The model under review builds one solid part; all positions refer to its coordinate system, in mm. A direction names the side the tool comes from. Round coordinates to 2 decimals unless told otherwise and drop trailing zeros. One line per item, written item: value. Start each with the question number.
1) Mouldability with a two-part tool opening along Y and no side actions: class faces 1 (the face through (-84.437, -39.217, 4.986)), 2 (the face through (-1, 1, 6)), 3 (the face through (-1, -75, 3)) as +Y half, -Y half, draft (parallel to the pull), parting line (faces both ways), or undercut.
2) Tool access review of faces 4 (the face through (84.73, -35.05, 1.97)), 5 (the face through (-84.437, 36.783, 4.986)): name each direction out of +Z, -Z, +X, -X, +Y, -Y from which nothing blocks a thin tool from reaching the whole face with its end or side.
3) Wall thickness on probe 1 along Y at (x, z) = (-82.85, 1.05); probe 2 along Y at (x, z) = (82.85, 4.5): over which ranges is each line inside the solid? List them lowest first.
4) For P1, Ø3.5, axis at x = -82, y = -37.5, coming from the -Z side, flat-tipped, find the tip position at first contact; note if it passes through.
from build123d import *

# Parameters (mm, degrees)
F0_W     = 200
F0_H     = 150
F0_R     = 3.5
F0_R_2   = 2
F1_DEPTH = 6
F2_DEPTH = 4


with BuildPart() as f1:
    # F0 (on Top) → F1 (new body)
    with BuildSketch(Plane.XY):
        Rectangle(F0_W, F0_H)
        with Locations((-82.85, -38)):
            Circle(F0_R, mode=Mode.SUBTRACT)
        with Locations((82.85, -38)):
            Circle(F0_R, mode=Mode.SUBTRACT)
        with Locations((-82.85, 38)):
            Circle(F0_R, mode=Mode.SUBTRACT)
        with Locations((82.85, 38)):
            Circle(F0_R, mode=Mode.SUBTRACT)
        with Locations((-82.85, 38)):
            Circle(F0_R)
        with Locations((-82.85, 38)):
            Circle(F0_R_2, mode=Mode.SUBTRACT)
        with Locations((82.85, -38)):
            Circle(F0_R)
        with Locations((82.85, -38)):
            Circle(F0_R_2, mode=Mode.SUBTRACT)
        with Locations((82.85, 38)):
            Circle(F0_R)
        with Locations((82.85, 38)):
            Circle(F0_R_2, mode=Mode.SUBTRACT)
        with Locations((-82.85, -38)):
            Circle(F0_R)
        with Locations((-82.85, -38)):
            Circle(F0_R_2, mode=Mode.SUBTRACT)
    extrude(amount=F1_DEPTH)

    # F0 (on Top) → F2 (cut)
    with BuildSketch(Plane.XY):
        with Locations((-82.85, 38)):
            Circle(F0_R)
        with Locations((-82.85, 38)):
            Circle(F0_R_2, mode=Mode.SUBTRACT)
        with Locations((82.85, 38)):
            Circle(F0_R)
        with Locations((82.85, 38)):
            Circle(F0_R_2, mode=Mode.SUBTRACT)
        with Locations((82.85, -38)):
            Circle(F0_R)
        with Locations((82.85, -38)):
            Circle(F0_R_2, mode=Mode.SUBTRACT)
        with Locations((-82.85, -38)):
            Circle(F0_R)
        with Locations((-82.85, -38)):
            Circle(F0_R_2, mode=Mode.SUBTRACT)
    extrude(amount=F2_DEPTH, mode=Mode.SUBTRACT)


solid = f1.part
Checked values:
1. face 1: undercut
1. face 2: draft
1. face 3: -Y half
2. face 4: -Z
2. face 5: +Z, -Z
3. probe 1: y = -75 to -41.5, -34.5 to 34.5, 41.5 to 75
3. probe 2: y = -75 to -40, -36 to 36, 40 to 75
4. P1: stops at z = 4
